Part model, mm, in its own coordinate system. A direction names the side the tool comes from. Give positions to 0.01 mm unless a question says otherwise; leave off trailing zeros. Write each loop counter-clockwise with the first axis right and the second up, starting at its lowest first coordinate (ties: lowest second). Pieces come first, ordered by that corner, then holes.
```python
from build123d import *

# Parameters (mm, degrees)
F_01_EIGHT_MILLIMETRE_TRACK_BLANK_DEPTH        = 8
F_02_LOWER_CAGE_TIE_LANDING_DEPTH              = 8
F_03_BUMP_END_SUPPORT_LANDING_DEPTH            = 8
F_04_START                                     = -0.1
S04_RELIEF_FOR_THE_SWEPT_FLOATING_GUID_R       = 45.5
F_04_RELIEF_FOR_THE_SWEPT_FLOATING_GUIDE_DEPTH = 8.2
F_05_START                                     = -0.1
F_05_CONCENTRIC_GUIDE_AND_TANGENT_STOP_F_DEPTH = 8.2
F_06_START                                     = -0.1
S06_SUPPORT_FASTENERS_R                        = 3.3
F_06_SUPPORT_FASTENERS_DEPTH                   = 8.2
F_07_START                                     = -0.1
S07_BUMP_END_SUPPORT_REGISTER_UNDERSID_R       = 5.06
F_07_BUMP_END_SUPPORT_REGISTER_UNDERSIDE_DEPTH = 1.35
F_08_START                                     = 4.5
S08_FLUSH_BUTTON_SCREW_COUNTERBORE_OUT_R       = 5.5
F_08_FLUSH_BUTTON_SCREW_COUNTERBORE_OUTB_DEPTH = 3.6


with BuildPart() as part:
    # S01 - Eight millimetre track blank → 01 - Eight millimetre track blank (new body)
    with BuildSketch(Plane.XY):
        with BuildLine():
            Line((25.527156043, -37.845565187), (42.69437818, -63.297018665))
            ThreePointArc((42.69437818, -63.297018665), (74.240443422, -17.82355353), (66.77721464, 37.015214506))
            Line((66.77721464, 37.015214506), (39.926389631, 22.131559164))
            ThreePointArc((39.926389631, 22.131559164), (44.388686866, -10.65678086), (25.527156043, -37.845565187))
        make_face()
    extrude(amount=F_01_EIGHT_MILLIMETRE_TRACK_BLANK_DEPTH)

    # S02 - Lower cage tie landing → 02 - Lower cage tie landing (add)
    with BuildSketch(Plane.XY):
        with BuildLine():
            Line((-1.286113116, -44.083049206), (34.568787274, -39.433085863))
            ThreePointArc((34.568787274, -39.433085863), (45.771851184, -48.063923541), (37.141013506, -59.266987451))
            Line((37.141013506, -59.266987451), (1.286113116, -63.916950794))
            ThreePointArc((1.286113116, -63.916950794), (-9.916950794, -55.286113116), (-1.286113116, -44.083049206))
        make_face()
    extrude(amount=F_02_LOWER_CAGE_TIE_LANDING_DEPTH)

    # S03 - Bump end support landing → 03 - Bump end support landing (add)
    with BuildSketch(Plane.XY):
        with BuildLine():
            Line((45.572351488, 20.615526776), (42.574781821, 26.253135379))
            ThreePointArc((42.574781821, 26.253135379), (47.123018152, 41.129746091), (61.999628864, 36.58150976))
            Line((61.999628864, 36.58150976), (64.997198531, 30.943901157))
            ThreePointArc((64.997198531, 30.943901157), (60.4489622, 16.067290445), (45.572351488, 20.615526776))
        make_face()
    extrude(amount=F_03_BUMP_END_SUPPORT_LANDING_DEPTH)

    # S04 - Relief for the swept floating guide barrels → 04 - Relief for the swept floating guide barrels (cut)
    with BuildSketch(Plane.XY.offset(F_04_START)):
        Circle(S04_RELIEF_FOR_THE_SWEPT_FLOATING_GUID_R)
    extrude(amount=F_04_RELIEF_FOR_THE_SWEPT_FLOATING_GUIDE_DEPTH, mode=Mode.SUBTRACT)

    # S05 - Concentric guide and tangent stop faces → 05 - Concentric guide and tangent stop faces (cut)
    with BuildSketch(Plane.XY.offset(F_05_START)):
        with BuildLine():
            Line((34.862224899, -39.454375867), (45.92013859, -51.968869257))
            ThreePointArc((45.92013859, -51.968869257), (66.319734826, -20.275977723), (67.130143118, 17.405929591))
            Line((67.130143118, 17.405929591), (50.9647013, 13.214451233))
            ThreePointArc((50.9647013, 13.214451233), (50.349445401, -15.393370254), (34.862224899, -39.454375867))
        make_face()
    extrude(amount=F_05_CONCENTRIC_GUIDE_AND_TANGENT_STOP_F_DEPTH, mode=Mode.SUBTRACT)

    # S06 - Support fasteners → 06 - Support fasteners (cut)
    with BuildSketch(Plane.XY.offset(F_06_START)):
        with Locations(Location((0, -54, 0), (0, 0, 180))):
            Circle(S06_SUPPORT_FASTENERS_R)
        with Locations(Location((52.287205343, 31.41732257, 0), (0, 0, 180))):
            Circle(S06_SUPPORT_FASTENERS_R)
    extrude(amount=F_06_SUPPORT_FASTENERS_DEPTH, mode=Mode.SUBTRACT)

    # S07 - Bump end support register underside → 07 - Bump end support register underside (cut)
    with BuildSketch(Plane.XY.offset(F_07_START)):
        with Locations(Location((52.287205343, 31.41732257, 0), (0, 0, 180))):
            Circle(S07_BUMP_END_SUPPORT_REGISTER_UNDERSID_R)
    extrude(amount=F_07_BUMP_END_SUPPORT_REGISTER_UNDERSIDE_DEPTH, mode=Mode.SUBTRACT)

    # S08 - Flush button screw counterbore outboard → 08 - Flush button screw counterbore outboard (cut)
    with BuildSketch(Plane.XY.offset(F_08_START)):
        with Locations(Location((52.287205343, 31.41732257, 0), (0, 0, 180))):
            Circle(S08_FLUSH_BUTTON_SCREW_COUNTERBORE_OUT_R)
    extrude(amount=F_08_FLUSH_BUTTON_SCREW_COUNTERBORE_OUTB_DEPTH, mode=Mode.SUBTRACT)


solid = part.part
```
1) Saw through at C-C, the plane z = 3. Write the cut outline in (x, y).
Answers follow:
outline: (-4.83, -45.24) arc R10 ccw to (1.29, -63.92) - (37.14, -59.27) arc R10 ccw to (39.55, -58.64) - (42.69, -63.3) arc R76.35 ccw to (66.78, 37.02) - (62.91, 34.87) - (62, 36.58) arc R11 ccw to (42.57, 26.25) - (43.66, 24.2) - (39.93, 22.13) arc R45.65 cw to (25.53, -37.85) - (27.24, -40.38) - (18.66, -41.5) arc R45.5 cw to start; hole circle Ø6.6 at (0, -54); hole (34.86, -39.45) - (45.92, -51.97) arc R69.35 ccw to (67.13, 17.41) - (50.96, 13.21) arc R52.65 cw to start; hole circle Ø6.6 at (52.29, 31.42)
2) Pin check, flat tips, straight feed: pin 1 Ø2 at (x, z) = (18, 1.5) entering from -Y; pin 2 Ø2 at (y, z) = (-2, 2.5) entering from +X; pin 3 Ø2 at (y, z) = (-31, 1) entering from -X; pin 4 Ø5.5 at (x, y) = (0, -54) entering from -Z. Stop position of each tip, or through.
Answers follow:
pin 1: stops at y = -61.88
pin 2: stops at x = 76.34
pin 3: stops at x = 32.56
pin 4: passes through
3) Saw through at B-B, the plane y = -11. Write the cut outline in (x, z), then the cut area to 3 significant figures.
Answers follow:
outline: (44.3, 0) - (51.49, 0) - (51.49, 8) - (44.3, 8) - close; (68.47, 0) - (75.55, 0) - (75.55, 8) - (68.47, 8) - close
area: 114 mm2
4) Saw through at D-D, the plane x = 22.5. Write the cut outline in (y, z), then the cut area to 3 significant figures.
Answers follow:
outline: (-61.17, 0) - (-41, 0) - (-41, 8) - (-61.17, 8) - close
area: 161 mm2
5) Wall check: L1, parallel to Y at x = 53.5, z = 6.25; L2, parallel to Y at x = 64, z = 4.5; L3, parallel to X at y = -46.5, z = 3.5. Give the ranges that are in metal, low to high.
Answers follow:
L1: y = -54.47 to -44.13, 13.87 to 26.05, 36.78 to 42.35
L2: y = -41.63 to -26.71, 16.59 to 35.48
L3: x = -6.61 to 41.09, 51.45 to 60.56
6) 3-axis set-ups, long thin cutter, end or side, ignore diameter. For faces 4 (the face through (52, 35, 1.25)), 5 (the face through (52, 35, 4.5)), 6 (the face through (19.46, -61.56, 3.94)), 7 (the face through (59.16, 15.34, 3.94)): which of +Z, -Z, +X, -X, +Y, -Y reach the whole face in a straight line?
Answers follow:
face 4: -Z
face 5: +Z
face 6: +Z, -Z, -Y
face 7: +Z, -Z
7) Saw through at A-A, the plane x = 0. Write the cut outline in (y, z), then the cut area to 3 significant figures.
Answers follow:
outline: (-64, 0) - (-57.3, 0) - (-57.3, 8) - (-64, 8) - close; (-50.7, 0) - (-45.5, 0) - (-45.5, 8) - (-50.7, 8) - close
area: 95.2 mm2
8) Two-plate mould, pull along Y, no slides. Class faces 1 (the face through (43, -22, 8)), 2 (the face through (64.87, 35.96, 3.94)), 3 (the face through (41.82, 23.18, 3.94)): +Y half, -Y half, draft (parallel to the pull), parting line (faces both ways), or undercut.
Answers follow:
face 1: draft
face 2: +Y half
face 3: undercut
